The listing builds one solid part. Answer for the finished solid, in the listing's coordinates (mm). A direction names the side the tool comes from. Round coordinates to 2 decimals unless told otherwise and drop trailing zeros. Order: outer loops, then holes, each group sorted by start corner. A loop starts at its lowest first (then second) coordinate and runs counter-clockwise, first axis right, second up. Notation, with made-up numbers: (25, 28) -> (53, 28) arc R19 cw to (53, 55) -> close; hole circle Ø7 at (16, 40). An arc over 180 degrees is marked (long way). Answer in a Markdown table with one row per item. Add a question column.
```python
from build123d import *

# Parameters (mm, degrees)
F0_W     = 50.8
F0_H     = 50.8
F1_DEPTH = 50.8
F2_R     = 12.7
F3_DEPTH = 25.4
F4_R     = 5.08
F5_R     = 5.08
F6_W     = 30.48
F6_H     = 30.48
F7_DEPTH = 127
F8_R     = 5.08


with BuildPart() as f1:
    # F0 (on Top) → F1 (new body)
    with BuildSketch(Plane.XY):
        with Locations((25.4, 25.4)):
            Rectangle(F0_W, F0_H)
    extrude(amount=F1_DEPTH)

    # F2 (on face) → F3 (cut)
    with BuildSketch(Plane.XY.offset(50.8)):
        with Locations((25.4, 25.4)):
            Circle(F2_R)
    extrude(amount=-F3_DEPTH, mode=Mode.SUBTRACT)

    # F4
    f4_edges = [f1.edges().sort_by_distance(p)[0] for p in [
        (25.4, 50.8, 50.8),
        (50.8, 25.4, 50.8),
        (25.4, 0, 50.8),
        (0, 25.4, 50.8),
        (50.8, 0, 25.4),
        (50.8, 50.8, 25.4),
        (50.8, 25.4, 0),
        (0, 0, 25.4),
        (25.4, 0, 0),
        (0, 50.8, 25.4),
        (0, 25.4, 0),
        (25.4, 50.8, 0),
    ]]
    fillet(f4_edges, radius=F4_R)

    # F5
    f5_edges = [f1.edges().sort_by_distance(p)[0] for p in [
        (12.7, 25.4, 25.4),
        (12.7, 25.4, 50.8),
    ]]
    fillet(f5_edges, radius=F5_R)

    # F6 (on face) → F7 (join)
    with BuildSketch(Plane.YZ.offset(50.8)):
        with Locations((25.4, 25.4)):
            Rectangle(F6_W, F6_H)
    extrude(amount=F7_DEPTH)

    # F8
    f8_edges = [f1.edges().sort_by_distance(p)[0] for p in [
        (114.3, 10.16, 10.16),
        (114.3, 40.64, 40.64),
        (114.3, 40.64, 10.16),
        (177.8, 25.4, 10.16),
        (177.8, 40.64, 25.4),
        (177.8, 25.4, 40.64),
        (177.8, 10.16, 25.4),
    ]]
    fillet(f8_edges, radius=F8_R)


solid = f1.part
```
Item 1: The part is cut by section B-B, the plane x = 136.5. Give the vertices of the cut face in (y, z).
Item 2: A tool of negligible diameter and unlimited length cuts with its end or side. For faces 1 (the face through (112.613, 39.112, 39.191)), 2 (the face through (111, 25, 10.16)), 3 (the face through (111, 23, 40.64)), from which of +Z, -Z, +X, -X, +Y, -Y can it reach the whole face along a straight path? Write none if from no direction.
Item 3: The part is cut by section A-A, the plane y = 25.4. Give the vertices of the cut face in (x, z).
Item 4: Find the intervals of material crossed by probe 1 along X at (y, z) = (25, 41); probe 2 along X at (y, z) = (25, 36), in increasing order. Write a range as [from, to].
Item 5: Flat-ended cylindrical pins translate along their axes: P1, Ø6, axis at x = 82.5, y = 29.5, coming from the -Z side; P2, Ø12, axis at x = 153, z = 7, coming from the +Y side; P3, Ø22.5, axis at x = 119.5, z = 24, coming from the +Y side. Find the tip coordinate at first contact, or state that the pin passes through.
Item 6: The part is cut by section D-D, the plane z = 33.5. Give the vertices of the cut face in (x, y), and give its area (3 significant figures).
Item 7: For a pull along Y with two mould halves and no side action, classify faces 4 (the face through (25.684, 1.449, 49.272)), 5 (the face through (25, 26, 25.4)), 6 (the face through (25.684, 49.351, 49.272)), 7 (the face through (0, 25, 25)) as released by +Y, released by -Y, zero draft, split by the parting line, or undercut.
Item 8: The part is cut by section C-C, the plane z = 18. Give the vertices of the cut face in (x, y).
Resolved:
| question | item | result |
|---|---|---|
| 1 | outline | (10.16, 15.24) arc R5.08 ccw to (15.24, 10.16) -> (35.56, 10.16) arc R5.08 ccw to (40.64, 15.24) -> (40.64, 35.56) arc R5.08 ccw to (35.56, 40.64) -> (10.16, 40.64) -> close |
| 2 | face 1 | +Z, +X, +Y |
| 2 | face 2 | -Z, +X, +Y, -Y |
| 2 | face 3 | +Z, +X, +Y, -Y |
| 3 | outline | (0, 5.08) arc R5.08 ccw to (5.08, 0) -> (45.72, 0) arc R5.08 ccw to (50.8, 5.08) -> (50.8, 10.16) -> (172.72, 10.16) arc R5.08 ccw to (177.8, 15.24) -> (177.8, 35.56) arc R5.08 ccw to (172.72, 40.64) -> (50.8, 40.64) -> (50.8, 45.72) arc R5.08 ccw to (45.72, 50.8) -> (43.18, 50.8) arc R5.08 ccw to (38.1, 45.72) -> (38.1, 30.48) arc R5.08 cw to (33.02, 25.4) -> (17.78, 25.4) arc R5.08 cw to (12.7, 30.48) -> (12.7, 45.72) arc R5.08 ccw to (7.62, 50.8) -> (5.08, 50.8) arc R5.08 ccw to (0, 45.72) -> close |
| 4 | probe 1 | [0, 12.71], [38.09, 50.8] |
| 4 | probe 2 | [0, 12.71], [38.09, 177.78] |
| 5 | P1 | z = 10.16 |
| 5 | P2 | y = 40.12 |
| 5 | P3 | y = 40.64 |
| 6 | outline | (0, 5.08) arc R5.08 ccw to (5.08, 0) -> (45.72, 0) arc R5.08 ccw to (50.8, 5.08) -> (50.8, 10.16) -> (172.72, 10.16) arc R5.08 ccw to (177.8, 15.24) -> (177.8, 35.56) arc R5.08 ccw to (172.72, 40.64) -> (50.8, 40.64) -> (50.8, 45.72) arc R5.08 ccw to (45.72, 50.8) -> (5.08, 50.8) arc R5.08 ccw to (0, 45.72) -> close; hole circle Ø25.4 at (25.4, 25.4) |
| 6 | area | 5,910 mm2 |
| 7 | face 4 | released by -Y |
| 7 | face 5 | undercut |
| 7 | face 6 | released by +Y |
| 7 | face 7 | zero draft |
| 8 | outline | (0, 5.08) arc R5.08 ccw to (5.08, 0) -> (45.72, 0) arc R5.08 ccw to (50.8, 5.08) -> (50.8, 10.16) -> (172.72, 10.16) arc R5.08 ccw to (177.8, 15.24) -> (177.8, 35.56) arc R5.08 ccw to (172.72, 40.64) -> (50.8, 40.64) -> (50.8, 45.72) arc R5.08 ccw to (45.72, 50.8) -> (5.08, 50.8) arc R5.08 ccw to (0, 45.72) -> close |
